The model under review builds one solid part; all positions refer to its coordinate system, in mm. A direction names the side the tool comes from. Coordinates: 2 decimals unless noted, no trailing zeros. Loops run counter-clockwise (first coordinate to the right, second up) from the corner with the lowest first, then second, coordinate; pieces in that order, holes last. Notation, with made-up numbers: (-9, 80) -> (25, 80) arc R27 ccw to (25, 103) -> close; hole circle Ø9 at (-26.75, 82). An arc over 180 degrees is marked (long way). One line per question, with ' | ' between items. Start each with the question number.
Autodesk Fusion 360 part; units mm, degrees
sketch "Skizze1" plane through (0, 0, 0) normal (0, 0, 1) x (1, 0, 0)
  circle A0 centre (0, 0) radius 14
  circle A1 centre (0, 0) radius 15.5
  dimension "d1" = 28
  dimension "d2" = 31
extrude "Extrusion1" add sketch "Skizze1" along normal blind 521.6482 and the other way blind 150
equation "d3 = 40 mm + ( 13.25 * 36.2376 ) * 1 mm + 4.5 mm - 3 mm"

Autodesk Fusion 360 part; units mm, degrees
sketch "Skizze1" plane through (0, 0, 0) normal (0, 0, 1) x (1, 0, 0)
  circle A0 centre (0, 0) radius 200
  circle A1 centre (0, 0) radius 15.7
  circle A2 centre (0, 0) radius 54.873
  line L0 (50.553, -4.32) -> (50.553, 4.32)
  circle A3 centre (50.553, -4.32) radius 1.3
  circle A4 centre (59.193, -4.32) radius 1.3
  line L1 (50.553, -4.32) -> (59.193, 4.32) construction
  line L2 (50.553, 4.32) -> (59.193, 4.32)
  line L3 (59.193, -4.32) -> (50.553, 4.32) construction
  line L4 (59.193, 4.32) -> (59.193, -4.32)
  circle A5 centre (50.553, 4.32) radius 1.3
  circle A6 centre (54.873, 0) radius 2.25
  line L5 (59.193, -4.32) -> (50.553, -4.32)
  circle A7 centre (59.193, 4.32) radius 1.3
  circle A8 centre (-54.873, 0) radius 3.1
  circle A9 centre (38.8011, 38.8011) radius 3.1
  circle A10 centre (0, 54.873) radius 3.1
  circle A11 centre (-38.8011, 38.8011) radius 3.1
  circle A12 centre (-38.8011, -38.8011) radius 3.1
  circle A13 centre (0, -54.873) radius 3.1
  circle A14 centre (38.8011, -38.8011) radius 3.1
  point P0 (54.873, 0)
  point P1 (54.873, 0)
  dimension "d1" = 400
  dimension "d2" = 31.4
  dimension "d3" = 109.746
  dimension "d6" = 4.5
  dimension "d7" = 8.64
  dimension "d8" = 8.64
  dimension "d9" = 2.6
  dimension "d10" = 2.6
  dimension "d11" = 2.6
  dimension "d12" = 2.6
  dimension "d13" = 6.2
  dimension "d15" = 270
extrude "Extrusion1" add sketch "Skizze1" along normal blind 1.5 contours A0 | A2 L0 A3 L2 A5 A6 L5 | A2 A4 L2 L4 A6 L5 A7 | A2 L0 A3 L2 A5 L5 A8 A9 A10 A11 A12 A13 A14
1) Wall thickness on L1, parallel to X at y = 4.32, z = 1.1; L2, parallel to X at y = 11.5, z = -33; L3, parallel to Y at x = -33, z = 431: over which ranges is each line inside the solid? List them lowest first.
2) Insertion check: pin 1 Ø10 at (y, z) = (-110.5, 257.5) entering from +X; pin 2 Ø1 at (x, z) = (72, 130) entering from +Y; pin 3 Ø3 at (x, y) = (50.553, -4.32) entering from -Z; pin 4 Ø10 at (x, y) = (38.8, 38.8) entering from +Z. Each pin has a flat end and moves straight along its axis. Give the tip position at first contact, or say it passes through.
3) Consider section A-A, the plane z = 346. Write out the cut boundary in (x, y).
4) Consider section C-C, the plane y = 81.5. Write out the cut boundary in (x, z).
5) Consider section B-B, the plane x = 155. Write out the cut boundary in (y, z).
6) Machinability: for faces 1 (the face through (-20.76, -50.794, 257.933)), 2 (the face through (42, -42, 521.648)), 3 (the face through (21.237, 50.597, -73.95)), which of the approach directions +Z, -Z, +X, -X, +Y, -Y give a long, thin tool a straight path to every point of the face, cutting with its end or side? Answer none if there is none.
7) Mouldability with a two-part tool opening along Y and no side actions: class faces 4 (the face through (0, 0, 521.648)), 5 (the face through (50.36, -21.79, -73.95)), 6 (the face through (190.764, -60.075, 181.123)) as +Y half, -Y half, draft (parallel to the pull), parting line (faces both ways), or undercut.
Filled sheet:
1) L1: -199.95 to 49.25, 51.85 to 57.89, 60.49 to 199.95 | L2: -199.67 to -53.65, -10.69 to 10.69, 53.65 to 199.67 | L3: -197.26 to -43.84, 43.84 to 197.26
2) pin 1: x = 169.91 | pin 2: y = 186.78 | pin 3: z = 0 | pin 4: z = 521.65
3) outline: circle Ø400 at (0, 0); circle Ø31.4 at (0, 0); hole (-54.79, -3.1) arc R54.87 ccw to (-40.93, -36.55) arc R3.1 ccw (long way) to (-36.55, -40.93) arc R54.87 ccw to (-3.1, -54.79) arc R3.1 ccw (long way) to (3.1, -54.79) arc R54.87 ccw to (36.55, -40.93) arc R3.1 ccw (long way) to (40.93, -36.55) arc R54.87 ccw to (54.7, -4.32) -> (57.89, -4.32) arc R1.3 ccw (long way) to (59.19, -3.02) -> (59.19, 3.02) arc R1.3 ccw (long way) to (57.89, 4.32) -> (54.7, 4.32) arc R54.87 ccw to (40.93, 36.55) arc R3.1 ccw (long way) to (36.55, 40.93) arc R54.87 ccw to (3.1, 54.79) arc R3.1 ccw (long way) to (-3.1, 54.79) arc R54.87 ccw to (-36.55, 40.93) arc R3.1 ccw (long way) to (-40.93, 36.55) arc R54.87 ccw to (-54.79, 3.1) arc R3.1 ccw (long way) to start
4) outline: (-182.64, -150) -> (182.64, -150) -> (182.64, 521.65) -> (-182.64, 521.65) -> close
5) outline: (-126.39, -150) -> (126.39, -150) -> (126.39, 521.65) -> (-126.39, 521.65) -> close
6) face 1: +Z | face 2: +Z, +X, -X, +Y, -Y | face 3: -Z
7) face 4: draft | face 5: undercut | face 6: parting line
